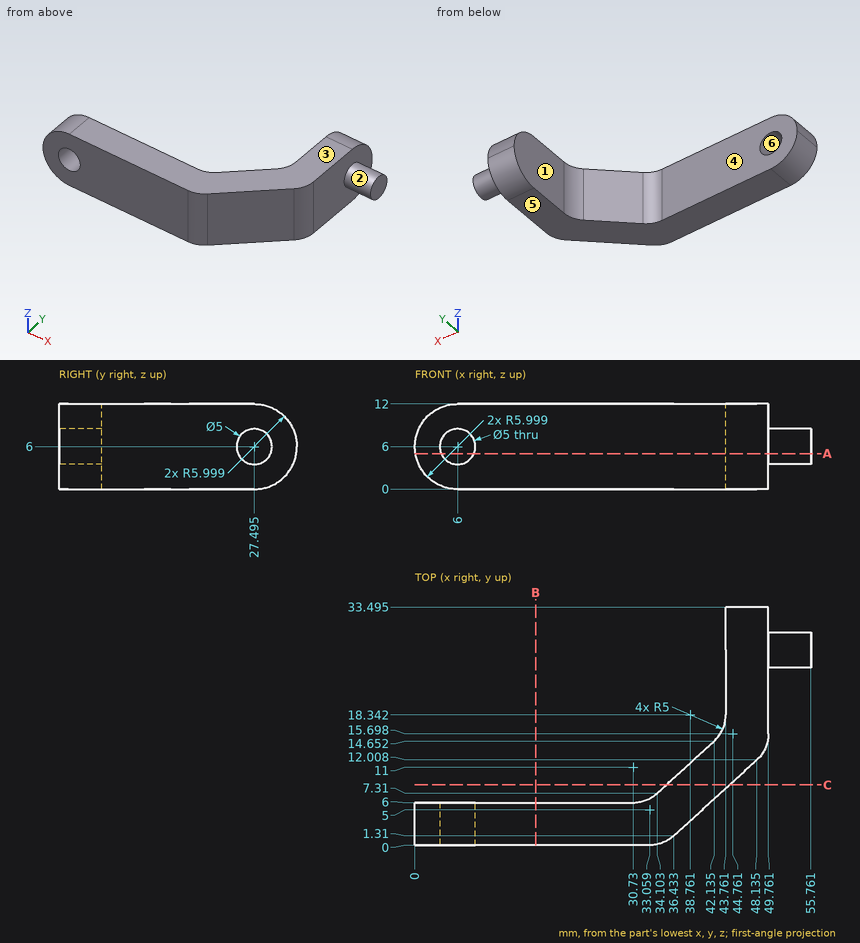
Job drawing, mm, ordinate dimensions from the low corner. One solid piece. A direction names the side the tool comes from. Give positions to 0.01 mm unless a question says otherwise; leave off trailing zeros. Order: outer loops, then holes, each group sorted by start corner. A loop starts at its lowest first (then second) coordinate and runs counter-clockwise, first axis right, second up. Notation, with made-up numbers: (15.5, 77) -> (20.5, 77) arc R19 cw to (20.5, 110) -> close; hole circle Ø6 at (-12.5, 27). An arc over 180 degrees is marked (long way). Return JSON: item names as keys, results as strings.
Q1. Saw through at A-A (z = 5). Write the cut outline in (x, y) (1 decimal), then the cut area to 3 significant figures.
Working result:
{"outline": "(0.1, 0) -> (3.7, 0) -> (3.7, 6) -> (0.1, 6) -> close; (8.3, 0) -> (33.1, 0) arc R5 ccw to (36.4, 1.3) -> (48.1, 12) arc R5 ccw to (49.8, 15.7) -> (49.8, 25.2) -> (55.8, 25.2) -> (55.8, 29.8) -> (49.8, 29.8) -> (49.8, 33.4) -> (43.8, 33.4) -> (43.8, 18.3) arc R5 cw to (42.1, 14.7) -> (34.1, 7.3) arc R5 cw to (30.7, 6) -> (8.3, 6) -> close", "area": "419 mm²"}
Q2. Which spindle directions (+Z, -Z, +X, -X, +Y, -Y) get a long thin tool onto all of the face, cutting with end or side? Do the marked faces 1, 2 and 3. Say none if no direction does.
Working result:
{"face 1": "+Z, -Z, -X, +Y", "face 2": "+X", "face 3": "+Z, +X, -X, +Y, -Y"}
Q3. Saw through at B-B (x = 17). Write the cut outline in (y, z), then the cut area to 3 significant figures.
Working result:
{"outline": "(0, 0) -> (6, 0) -> (6, 12) -> (0, 12) -> close", "area": "72.0 mm²"}
Q4. Flat gauge pins, fed straight in: pin 1 (6 mm diameter, centred on y = 23.5, z = 4.5, fed in from +X); pin 2 (6 mm diameter, centred on y = 9, z = 5, fed in from +X) (1 decimal); pin 3 (2 mm diameter, centred on x = 37, z = 2, fed in from +Y). Where does each tip first touch, or does it go through?
Working result:
{"pin 1": "x = 55.76", "pin 2": "x = 48.1", "pin 3": "y = 10.87"}
Q5. Drill centre lines: line 1 (Z direction, x = 6, y = 4.25); line 2 (Y direction, x = 29.5, z = 4); line 3 (X direction, y = 28, z = 8.25). Where is each one in solid material? Low to high.
Working result:
{"line 1": "0 to 3.5, 8.5 to 12", "line 2": "0 to 6", "line 3": "43.76 to 55.76"}
Q6. Mould opens along Z. For the marked faces 4, 5 and 6 say: pulls with the +Z half, pulls with the -Z half, needs draft (parallel to the pull), parting line crosses it, or undercut.
Working result:
{"face 4": "needs draft", "face 5": "pulls with the -Z half", "face 6": "undercut"}
Q7. Saw through at C-C (y = 8.5). Write the cut outline in (x, z) (1 decimal).
Working result:
{"outline": "(35.4, 0) -> (44.3, 0) -> (44.3, 12) -> (35.4, 12) -> close"}
